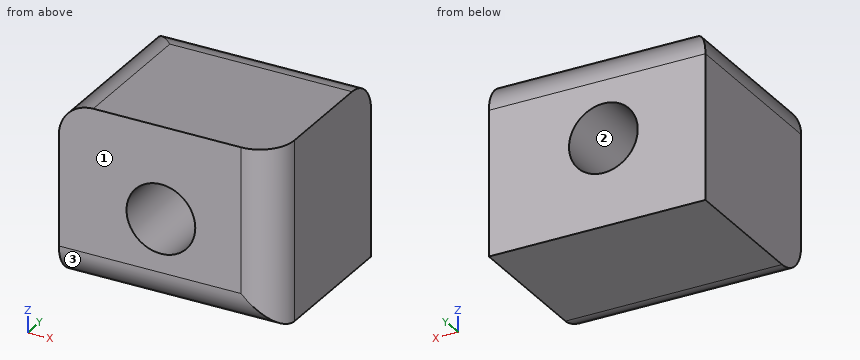
from build123d import *

# Parameters (mm, degrees)
F0_W     = 31.984137
F0_H     = 26.448421
F0_R     = 5.08
F1_DEPTH = 12.7
F2_R     = 5.08


with BuildPart() as f1:
    # F0 (on Front) → F1 (new body, symmetric)
    with BuildSketch(Plane.XZ):
        with Locations((-38.442476, 39.980176)):
            Rectangle(F0_W, F0_H)
        with Locations((-39.365098, 39.672639)):
            Circle(F0_R, mode=Mode.SUBTRACT)
    extrude(amount=F1_DEPTH, both=True)

    # F2
    f2_edges = [f1.edges().sort_by_distance(p)[0] for p in [
        (-38.442477, 12.7, 53.204387),
        (-54.434545, 0, 53.204387),
        (-22.450408, -12.7, 39.980177),
        (-38.442477, -12.7, 26.755966),
    ]]
    fillet(f2_edges, radius=F2_R)


solid = f1.part
Can you work these out from the model? Positions are in its coordinate system, mm. Face numbers are marked on the shaded views. Round coordinates to 2 decimals unless told otherwise and drop trailing zeros. Loops run counter-clockwise (first coordinate to the right, second up) from the corner with the lowest first, then second, coordinate; pieces in that order, holes last. Notation, with made-up numbers: (89.5, 72) - (123.5, 72) arc R37 ccw to (123.5, 111) - close; hole circle Ø5 at (20.25, 17). An arc over 180 degrees is marked (long way). Use CSV: the item, a comma, the result in double quotes. Start each with the question number.
1) If we section it at B-B on x = -42.5: Write out the boundary of the cut face in (y, z), plus the area to 3 significant figures.
2) If we section it at D-D on x = -36: Write out the boundary of the cut face in (y, z).
3) We'd pull the mould along Z, two halves only. Please class the marked faces 1, 2 and 3: released by +Z, released by -Z, zero draft, split by the parting line, or undercut.
4) Please list where these lines run through material, in increasing order: probe 1 along X at (y, z) = (9.75, 43); probe 2 along X at (y, z) = (-10.75, 39.75); probe 3 along Z at (x, y) = (-37, -2.5). Write a range as [from, to].
5) If we section it at C-C on y = 6.5: Write out the boundary of the cut face in (x, z).
6) If we section it at A-A on z = 38.5: Write out the boundary of the cut face in (x, y).
Geometry results:
1,outline,"(-12.7, 31.84) arc R5.08 ccw to (-7.62, 26.76) - (12.7, 26.76) - (12.7, 35.68) - (-12.7, 35.68) - close; (-12.7, 43.67) - (12.7, 43.67) - (12.7, 48.12) arc R5.08 ccw to (7.62, 53.2) - (-12.7, 53.2) - close"
1,area,"458 mm2"
2,outline,"(-12.7, 31.84) arc R5.08 ccw to (-7.62, 26.76) - (12.7, 26.76) - (12.7, 35.87) - (-12.7, 35.87) - close; (-12.7, 43.48) - (12.7, 43.48) - (12.7, 48.12) arc R5.08 ccw to (7.62, 53.2) - (-12.7, 53.2) - close"
3,face 1,"zero draft"
3,face 2,"undercut"
3,face 3,"released by -Z"
4,probe 1,"x = [-54.43, -43.2], [-35.53, -22.45]"
4,probe 2,"x = [-54.43, -44.44], [-34.29, -23.53]"
4,probe 3,"z = [26.76, 35.18], [44.17, 53.2]"
5,outline,"(-54.43, 26.76) - (-22.45, 26.76) - (-22.45, 53.2) - (-49.35, 53.2) arc R5.08 ccw to (-54.43, 48.12) - close; hole circle Ø10.16 at (-39.37, 39.67)"
6,outline,"(-54.43, -12.7) - (-44.31, -12.7) - (-44.31, 12.7) - (-54.43, 12.7) - close; (-34.42, -12.7) - (-27.53, -12.7) arc R5.08 ccw to (-22.45, -7.62) - (-22.45, 12.7) - (-34.42, 12.7) - close"
